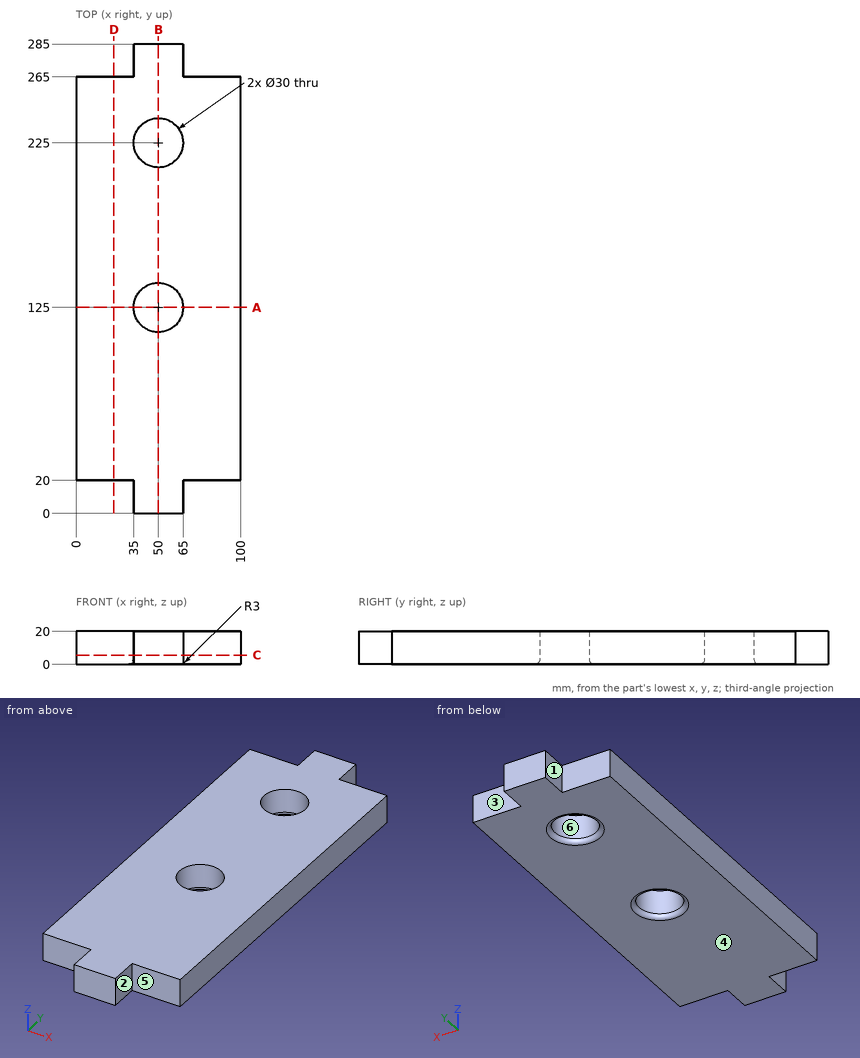
Input: dimensioned drawing with shaded views. Units: mm. Origin: part minimum x, y, z. A direction names the side the tool comes from. Round coordinates to 2 decimals unless told otherwise and drop trailing zeros. Loops run counter-clockwise (first coordinate to the right, second up) from the corner with the lowest first, then second, coordinate; pieces in that order, holes last. Notation, with made-up numbers: M 8,46 L 13,46 A11 cw 13,54 Z; hole C 34.5,75.5 d3. An arc over 180 degrees is marked long. Return JSON: item names as keys, results as strings. Group by question number.
1. Section query D-D on x = 23. Output: boundary loops of the cut face in (y, z).
2. Section query B-B on x = 50. Output: boundary loops of the cut face in (y, z), and give its area (3 significant figures).
3. Section query A-A on y = 125. Output: boundary loops of the cut face in (x, z), and give its area (3 significant figures).
4. Mould query, pull axis Y, two halves, no side actions, for the marked faces 4, 5 and 6. Classes: released by +Y, released by -Y, zero draft, split by the parting line, or undercut.
5. Section query C-C on z = 5.5. Output: boundary loops of the cut face in (x, y).
6. Pin query (flat end, axial travel): pin 1 (10 mm diameter, centred on x = 76.5, z = 7, fed in from +Y); pin 2 (10 mm diameter, centred on x = 21, z = 14, fed in from -Y); pin 3 (6 mm diameter, centred on y = 271, z = 5, fed in from +X); pin 4 (18 mm diameter, centred on x = 50, y = 125, fed in from +Z). Return the tip coordinate at first contact, or that it passes through.
7. Material intervals for line 1 along Y through (x, z) = (50, 15.25); line 2 along Y through (x, z) = (40, 2.75); line 3 along Y through (x, z) = (69.5, 18), sorted ascending. Write a range as from..to.
8. Reachability of the marked faces 1, 2 and 3 from +Z, -Z, +X, -X, +Y, -Y: full face, straight path, thin tool, end or side. Return the list, or none.
Checks:
{
 "1": {"outline": "M 20,0 L 265,0 L 265,20 L 20,20 Z"},
 "2": {"outline": "M 0,0 L 107,0 A3 ccw 110,3 L 110,20 L 0,20 Z; M 140,3 A3 ccw 143,0 L 207,0 A3 ccw 210,3 L 210,20 L 140,20 Z; M 240,3 A3 ccw 243,0 L 285,0 L 285,20 L 240,20 Z", "area": "4,490 mm²"},
 "3": {"outline": "M 0,0 L 32,0 A3 ccw 35,3 L 35,20 L 0,20 Z; M 65,3 A3 ccw 68,0 L 100,0 L 100,20 L 65,20 Z", "area": "1,400 mm²"},
 "4": {"face 4": "zero draft", "face 5": "released by -Y", "face 6": "undercut"},
 "5": {"outline": "M 0,20 L 35,20 L 35,0 L 65,0 L 65,20 L 100,20 L 100,265 L 65,265 L 65,285 L 35,285 L 35,265 L 0,265 Z; hole C 50,125 d30; hole C 50,225 d30"},
 "6": {"pin 1": "stops at y = 265", "pin 2": "stops at y = 20", "pin 3": "stops at x = 65", "pin 4": "passes through"},
 "7": {"line 1": "y = 0..110, 140..210, 240..285", "line 2": "y = 0..113.81, 136.19..213.81, 236.19..285", "line 3": "y = 20..265"},
 "8": {"face 1": "+Z, -Z, -X, +Y", "face 2": "+Z, -Z, +X, -Y", "face 3": "+Z, -Z, +X, +Y"}
}
